from build123d import *

# Parameters (mm, degrees)
SKETCH1_W           = 58.928
SKETCH1_H           = 31.75
BOSS_EXTRUDE1_DEPTH = 32.512
CUT_EXTRUDE1_DEPTH  = 12.7
SKETCH4_W           = 23.368
SKETCH4_H           = 9.652
CUT_EXTRUDE2_DEPTH  = 11.176


with BuildPart() as part:
    # Sketch1 → Boss-Extrude1 (new body)
    with BuildSketch(Plane(origin=(0, 0, 0), x_dir=(1, 0, 0), z_dir=(0, 1, 0))):
        with Locations((29.464, 15.875)):
            Rectangle(SKETCH1_W, SKETCH1_H)
    extrude(amount=BOSS_EXTRUDE1_DEPTH)

    # Sketch3 → Cut-Extrude1 (cut)
    with BuildSketch(Plane.XY):
        Polygon((26.924, 32.512), (58.928, 11.1252), (58.928, 32.512), align=None)
    extrude(amount=-CUT_EXTRUDE1_DEPTH, mode=Mode.SUBTRACT)

    # Sketch4 → Cut-Extrude2 (cut)
    with BuildSketch(Plane(origin=(0, 32.512, 0), x_dir=(1, 0, 0), z_dir=(0, 1, 0))):
        with Locations((11.684, 26.924)):
            Rectangle(SKETCH4_W, SKETCH4_H)
    extrude(amount=-CUT_EXTRUDE2_DEPTH, mode=Mode.SUBTRACT)


solid = part.part
The listing builds one solid part. Answer for the finished solid, in the listing's coordinates (mm). A direction names the side the tool comes from. Give positions to 0.01 mm unless a question says otherwise; leave off trailing zeros. Write each loop counter-clockwise with the first axis right and the second up, starting at its lowest first coordinate (ties: lowest second). Pieces come first, ordered by that corner, then holes.
1) A tool of negligible diameter and unlimited length cuts with its end or side. For faces 1 (the face through (50, 27, -12.7)), 2 (the face through (0, 16, -16)), 3 (the face through (12, 27, -22.098)), from which of +Z, -Z, +X, -X, +Y, -Y can it reach the whole face along a straight path? Write none if from no direction.
2) Given P1, Ø3.5, axis at x = 15.5, y = 27.5, coming from the -Z side; P2, Ø6.5, axis at x = 51, y = 20.5, coming from the +Z side; P3, Ø5, axis at x = 8.5, z = -25, coming from the +Y side, each flat-ended and moving along its own axis, determine where each tip first touches the part or whether it passes through.
3) Section B-B (z = -10) is taken. Write down the section's boundary in (x, y).
4) Find the intervals of material crossed by L1, parallel to Z at x = 39.5, y = 30.5; L2, parallel to X at y = 21.5, z = -26; L3, parallel to Z at x = 21, y = 28.5, in increasing order.
5) Section D-D (z = -25) is taken. Write down the section's boundary in (x, y).
6) Section A-A (x = 10) is taken. Write down the section's boundary in (y, z).
7) Section C-C (y = 29) is taken. Write down the section's boundary in (x, z), and give its area (3 significant figures).
Response:
1. face 1: +Z, +X, +Y
1. face 2: +Z, -Z, -X, +Y, -Y
1. face 3: -Z, -X, +Y
2. P1: stops at z = -22.1
2. P2: stops at z = -12.7
2. P3: stops at y = 21.34
3. outline: (0, 0) - (58.93, 0) - (58.93, 11.13) - (26.92, 32.51) - (0, 32.51) - close
4. L1: z = -31.75 to -12.7
4. L2: x = 23.37 to 58.93
4. L3: z = -22.1 to 0
5. outline: (0, 0) - (58.93, 0) - (58.93, 32.51) - (23.37, 32.51) - (23.37, 21.34) - (0, 21.34) - close
6. outline: (0, -31.75) - (21.34, -31.75) - (21.34, -22.1) - (32.51, -22.1) - (32.51, 0) - (0, 0) - close
7. outline: (0, -22.1) - (23.37, -22.1) - (23.37, -31.75) - (58.93, -31.75) - (58.93, -12.7) - (32.18, -12.7) - (32.18, 0) - (0, 0) - close
7. area: 1,310 mm2
